Model file for the job. Use its own axes, mm. Face numbers are marked on the shaded views. A direction names the side the tool comes from. Round coordinates to 2 decimals unless told otherwise and drop trailing zeros. Order: outer loops, then holes, each group sorted by start corner. A loop starts at its lowest first (then second) coordinate and runs counter-clockwise, first axis right, second up. Notation, with made-up numbers: (-24.75, -39) -> (-6.75, -39) arc R6 cw to (-6.75, -31) -> close; hole circle Ø5 at (44, -37.5). An arc over 180 degrees is marked (long way). Put each result on its own line as item: value. Start each with the question number.
Q1. 3-axis set-ups, long thin cutter, end or side, ignore diameter. For the marked faces 1, 2, 3 and 4: which of +Z, -Z, +X, -X, +Y, -Y reach the whole face in a straight line?
Q2. Cut at B-B, the plane y = 0. List the corners of the cut face in (x, z).
Q3. Flat gauge pins, fed straight in: P1, Ø2, axis at x = 21, y = -12, coming from the +Z side; P2, Ø3, axis at y = 38.5, z = 20, coming from the -X side; P3, Ø1.5, axis at x = 3, z = 7.5, coming from the -Y side. Where does each tip first touch, or does it go through?
Q4. Cut at C-C, the plane z = 35.5. List the corners of the cut face in (x, y).
Q5. Cut at A-A, the plane x = 0. List the corners of the cut face in (y, z).
Q6. Probe L1, parallel to X at y = 0, z = 23; L2, parallel to Y at x = 0, z = 26; L3, parallel to Y at x = -24, z = 26. List the from-to ranges inside material, lowest first.
Q7. Cut at D-D, the plane y = 34.5. List the corners of the cut face in (x, z).
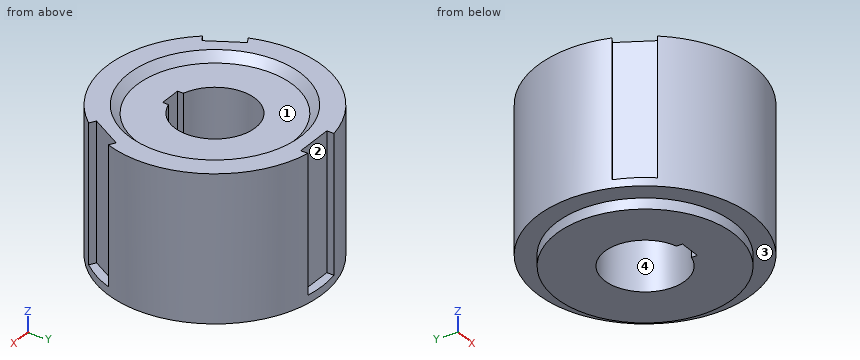
from build123d import *

# Parameters (mm, degrees)
ESQUISSE1_R             = 40
ESQUISSE1_R_2           = 33
ESQUISSE1_R_3           = 15
BOSS_EXTRU_1_DEPTH      = 58
ESQUISSE2_W             = 8
ESQUISSE2_H             = 3.3
ENL_V_MAT_EXTRU_1_DEPTH = 82.018516402
ENL_V_START             = -51
ENL_V_MAT_EXTRU_2_DEPTH = 51
ESQUISSE4_R             = 40
ESQUISSE4_R_2           = 33
ENL_V_MAT_EXTRU_3_DEPTH = 4


with BuildPart() as part:
    # Esquisse1 → Boss.-Extru.1 (new body)
    # profile 1 of 2: a face of its own
    with BuildSketch(Plane.XY):
        with Locations(Location((0, 0, 0), (0, 0, 180))):
            Circle(ESQUISSE1_R)
        Circle(ESQUISSE1_R_2, mode=Mode.SUBTRACT)
    # profile 2 of 2: a face of its own
    with BuildSketch(Plane.XY):
        Circle(ESQUISSE1_R_2)
        with Locations(Location((0, 0, 0), (0, 0, 180))):
            Circle(ESQUISSE1_R_3, mode=Mode.SUBTRACT)
    extrude(amount=BOSS_EXTRU_1_DEPTH)

    # Esquisse2 → Enlèv. mat.-Extru.1 (cut, through all)
    with BuildSketch(Plane.XY.offset(58)):
        with Locations((0, -15)):
            Rectangle(ESQUISSE2_W, ESQUISSE2_H)
    extrude(amount=-ENL_V_MAT_EXTRU_1_DEPTH, mode=Mode.SUBTRACT)

    # Esquisse3 → Enlèv. mat.-Extru.2 (cut)
    with BuildSketch(Plane.XY.offset(58).offset(ENL_V_START)):
        with BuildLine():
            Line((40.999452493, -15.588141165), (37.606451003, -13.629190841))
            ThreePointArc((37.606451003, -13.629190841), (34.641016151, -20), (30.606451003, -25.753546494))
            Line((30.606451003, -25.753546494), (33.999452493, -27.712496818))
            Line((33.999452493, -27.712496818), (40.999452493, -15.588141165))
        make_face()
        with BuildLine():
            ThreePointArc((30.606451003, -25.753546494), (34.641016151, -20), (37.606451003, -13.629190841))
            Line((37.606451003, -13.629190841), (35.28257981, -12.287503182))
            Line((35.28257981, -12.287503182), (28.28257981, -24.411858835))
            Line((28.28257981, -24.411858835), (30.606451003, -25.753546494))
        make_face()
        with BuildLine():
            ThreePointArc((-30.606451003, -25.753546494), (-34.641016151, -20), (-37.606451003, -13.629190841))
            Line((-37.606451003, -13.629190841), (-40.999452493, -15.588141165))
            Line((-40.999452493, -15.588141165), (-33.999452493, -27.712496818))
            Line((-33.999452493, -27.712496818), (-30.606451003, -25.753546494))
        make_face()
        with BuildLine():
            Line((-35.28257981, -12.287503182), (-37.606451003, -13.629190841))
            ThreePointArc((-37.606451003, -13.629190841), (-34.641016151, -20), (-30.606451003, -25.753546494))
            Line((-30.606451003, -25.753546494), (-28.28257981, -24.411858835))
            Line((-28.28257981, -24.411858835), (-35.28257981, -12.287503182))
        make_face()
        with BuildLine():
            ThreePointArc((7, 39.382737335), (0, 40), (-7, 39.382737335))
            Line((-7, 39.382737335), (-7, 36.699362017))
            Line((-7, 36.699362017), (7, 36.699362017))
            Line((7, 36.699362017), (7, 39.382737335))
        make_face()
        with BuildLine():
            Line((7, 43.300637983), (-7, 43.300637983))
            Line((-7, 43.300637983), (-7, 39.382737335))
            ThreePointArc((-7, 39.382737335), (0, 40), (7, 39.382737335))
            Line((7, 39.382737335), (7, 43.300637983))
        make_face()
    extrude(amount=ENL_V_MAT_EXTRU_2_DEPTH, mode=Mode.SUBTRACT)

    # Esquisse4 → Enlèv. mat.-Extru.3 (cut)
    with BuildSketch(Plane(origin=(0, 0, 0), x_dir=(-1, 0, 0), z_dir=(0, 0, -1))):
        Circle(ESQUISSE4_R)
        Circle(ESQUISSE4_R_2, mode=Mode.SUBTRACT)
    extrude(amount=-ENL_V_MAT_EXTRU_3_DEPTH, mode=Mode.SUBTRACT)

    # Esquisse7 → Enlèvement de matière-Révolution2 (revolve, cut)
    with BuildSketch(Plane(origin=(0, 0, 0), x_dir=(0, 0, -1), z_dir=(1, 0, 0)), mode=Mode.PRIVATE) as enl_vement_de_mati_re_r_volution2_sk:
        Polygon((-58, 32), (-55, 29), (-55, 0), (-58, 0), align=None)
    revolve(enl_vement_de_mati_re_r_volution2_sk.sketch.rotate(Axis((0, 0, 0), (0, 0, 1)), 90), axis=Axis((0, 0, 0), (0, 0, 1)), mode=Mode.SUBTRACT)


solid = part.part
Ans:
1. face 1: +Z
1. face 2: +Z, +Y
1. face 3: -Z
1. face 4: +Z, -Z
2. outline: (-40, 4) -> (-33, 4) -> (-33, 0) -> (-15, 0) -> (-15, 55) -> (-29, 55) -> (-32, 58) -> (-40, 58) -> close; (15, 0) -> (33, 0) -> (33, 4) -> (40, 4) -> (40, 58) -> (32, 58) -> (29, 55) -> (15, 55) -> close
3. P1: stops at z = 55
3. P2: stops at x = -15.2
3. P3: stops at y = -39.94
4. outline: (-37.61, -13.63) -> (-35.28, -12.29) -> (-28.28, -24.41) -> (-30.61, -25.75) arc R40 ccw to (30.61, -25.75) -> (28.28, -24.41) -> (35.28, -12.29) -> (37.61, -13.63) arc R40 ccw to (7, 39.38) -> (7, 36.7) -> (-7, 36.7) -> (-7, 39.38) arc R40 ccw to start; hole (-4, -16.65) -> (4, -16.65) -> (4, -14.46) arc R15 ccw (long way) to (-4, -14.46) -> close
5. outline: (-40, 4) -> (-33, 4) -> (-33, 0) -> (-16.65, 0) -> (-16.65, 55) -> (-29, 55) -> (-32, 58) -> (-40, 58) -> close; (15, 0) -> (33, 0) -> (33, 4) -> (40, 4) -> (40, 7) -> (36.7, 7) -> (36.7, 58) -> (32, 58) -> (29, 55) -> (15, 55) -> close
6. L1: x = -40 to -15, 15 to 40
6. L2: y = -40 to -16.65, 15 to 36.7
6. L3: y = -32 to 32
7. outline: (-20.24, 4) -> (20.24, 4) -> (20.24, 58) -> (-20.24, 58) -> close
